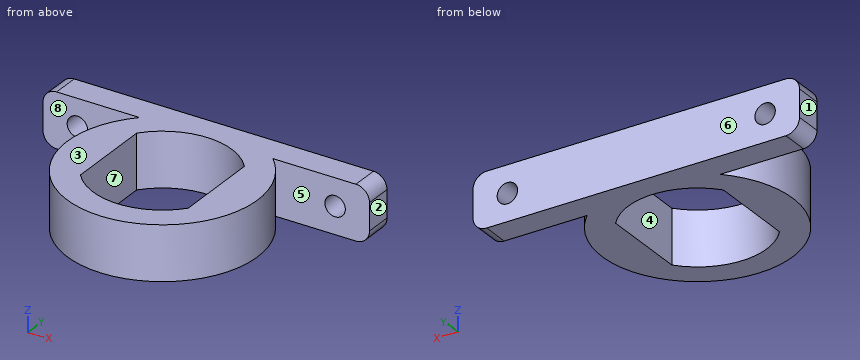
```python
from build123d import *

# Parameters (mm, degrees)
SALIENTE_EXTRUIR1_DEPTH = 8
CORTAR_EXTRUIR1_DEPTH   = 29.91366459
REDONDEO1_R             = 2
CROQUIS3_R              = 1.5
CORTAR_EXTRUIR2_DEPTH   = 35.871191548


with BuildPart() as part:
    # Croquis1 → Saliente-Extruir1 (new body)
    with BuildSketch(Plane.XY):
        with BuildLine():
            Line((0, 14), (-24, 14))
            Line((-24, 14), (-24, 10))
            Line((-24, 10), (-9.797958971, 10))
            ThreePointArc((-9.797958971, 10), (0, -14), (9.797958971, 10))
            Line((9.797958971, 10), (24, 10))
            Line((24, 10), (24, 14))
            Line((24, 14), (0, 14))
        make_face()
    extrude(amount=SALIENTE_EXTRUIR1_DEPTH)

    # Croquis2 → Cortar-Extruir1 (cut, through all)
    with BuildSketch(Plane.XY.offset(8)):
        with BuildLine():
            Line((-7.922081482, 6.425), (-7.922081482, -6.425))
            ThreePointArc((-7.922081482, -6.425), (0, -10.2), (7.922081482, -6.425))
            Line((7.922081482, -6.425), (7.922081482, 6.425))
            ThreePointArc((7.922081482, 6.425), (0, 10.2), (-7.922081482, 6.425))
        make_face()
    extrude(amount=-CORTAR_EXTRUIR1_DEPTH, mode=Mode.SUBTRACT)

    # Redondeo1
    redondeo1_edges = [part.edges().sort_by_distance(p)[0] for p in [
        (-24, 12, 8),
        (24, 12, 8),
        (-24, 12, 0),
        (24, 12, 0),
    ]]
    fillet(redondeo1_edges, radius=REDONDEO1_R)

    # Croquis3 → Cortar-Extruir2 (cut, through all)
    with BuildSketch(Plane(origin=(0, 10, 0), x_dir=(-1, 0, 0), z_dir=(0, -1, 0))):
        with Locations(Location((18.949489743, -4, 0), (0, 0, 90))):
            Circle(CROQUIS3_R)
        with Locations(Location((-18.949489743, -4, 0), (0, 0, 90))):
            Circle(CROQUIS3_R)
    extrude(amount=-CORTAR_EXTRUIR2_DEPTH, mode=Mode.SUBTRACT)


solid = part.part
```
The model under review builds one solid part; all positions refer to its coordinate system, in mm. Face numbers are marked on the shaded views. A direction names the side the tool comes from. Give positions to 0.01 mm unless a question says otherwise; leave off trailing zeros. Order: outer loops, then holes, each group sorted by start corner. A loop starts at its lowest first (then second) coordinate and runs counter-clockwise, first axis right, second up. Notation, with made-up numbers: (-28.5, 84.5) - (25.5, 84.5) arc R20 ccw to (25.5, 100.5) - close; hole circle Ø8 at (-8, 31.5). An arc over 180 degrees is marked (long way). Use CSV: the item, a comma, the result in double quotes. Start each with the question number.
Q1. We need section A-A, the plane z = 4. Write out the cut boundary in (x, y) (3 decimals), and give its area (3 significant figures).
Q2. We need section B-B, the plane y = 0. Write out the cut boundary in (x, z).
Q3. We need section C-C, the plane x = 0. Write out the cut boundary in (y, z), and give its area (3 significant figures).
Q4. We need section D-D, the plane z = 1.25. Write out the cut boundary in (x, y) (3 decimals), and give its area (3 significant figures).
Q5. To check wall thickness, follow line 1 along X through (y, z) = (12.45, 4); line 2 along Y through (x, z) = (-10, 0.75); line 3 along X through (y, z) = (0.75, 6). State the ranges of each line that lie inside material, in increasing order. Write a range as [from, to].
Q6. The part is to be moulded in two halves that separate along X. For the marked faces 1, 2, 3 and 4, say which applies: +X half, -X half, draft (parallel to the pull), parting line (faces both ways), or undercut.
Q7. Clearance check with flat-ended pins moving along their axes: pin 1 Ø1.8 at (x, z) = (18.95, 4) entering from +Y (3 decimals); pin 2 Ø3 at (y, z) = (1, 1.5) entering from +X; pin 3 Ø2.5 at (x, z) = (17, 5) entering from -Y; pin 4 Ø10 at (x, y) = (-7, -4.5) entering from -Z. State where each tip first meets the part, or that it passes through.
Q8. Tool access review of the marked faces 5, 6, 7 and 8: name each direction out of +Z, -Z, +X, -X, +Y, -Y from which nothing blocks a thin tool from reaching the whole face with its end or side.
Outcome:
1,outline,"(-24, 10) - (-20.449, 10) - (-20.449, 14) - (-24, 14) - close; (-17.449, 10) - (-9.798, 10) arc R14 ccw (long way) to (9.798, 10) - (17.449, 10) - (17.449, 14) - (-17.449, 14) - close; (20.449, 10) - (24, 10) - (24, 14) - (20.449, 14) - close; hole (-7.922, -6.425) arc R10.2 ccw to (7.922, -6.425) - (7.922, 6.425) arc R10.2 ccw to (-7.922, 6.425) - close"
1,area,"443 mm^2"
2,outline,"(-14, 0) - (-7.92, 0) - (-7.92, 8) - (-14, 8) - close; (7.92, 0) - (14, 0) - (14, 8) - (7.92, 8) - close"
3,outline,"(-14, 0) - (-10.2, 0) - (-10.2, 8) - (-14, 8) - close; (10.2, 0) - (14, 0) - (14, 8) - (10.2, 8) - close"
3,area,"60.8 mm^2"
4,outline,"(-23.854, 10) - (-9.798, 10) arc R14 ccw (long way) to (9.798, 10) - (23.854, 10) - (23.854, 14) - (-23.854, 14) - close; hole (-7.922, -6.425) arc R10.2 ccw to (7.922, -6.425) - (7.922, 6.425) arc R10.2 ccw to (-7.922, 6.425) - close"
4,area,"466 mm^2"
5,line 1,"x = [-24, -20.45], [-17.45, 17.45], [20.45, 24]"
5,line 2,"y = [-9.8, 9.8], [10, 14]"
5,line 3,"x = [-13.98, -7.92], [7.92, 13.98]"
6,face 1,"-X half"
6,face 2,"+X half"
6,face 3,"draft"
6,face 4,"undercut"
7,pin 1,"passes through"
7,pin 2,"stops at x = 14"
7,pin 3,"stops at y = 10"
7,pin 4,"stops at z = 0"
8,face 5,"+Z, -Z, +X"
8,face 6,"+Z, -Z, +X, -X, +Y"
8,face 7,"+Z, -Z"
8,face 8,"+Z, -Z, -X"
